Input: part model. Units: mm. Frame: model coordinates. Coordinates: 2 decimals unless noted, no trailing zeros. Loops run counter-clockwise (first coordinate to the right, second up) from the corner with the lowest first, then second, coordinate; pieces in that order, holes last.
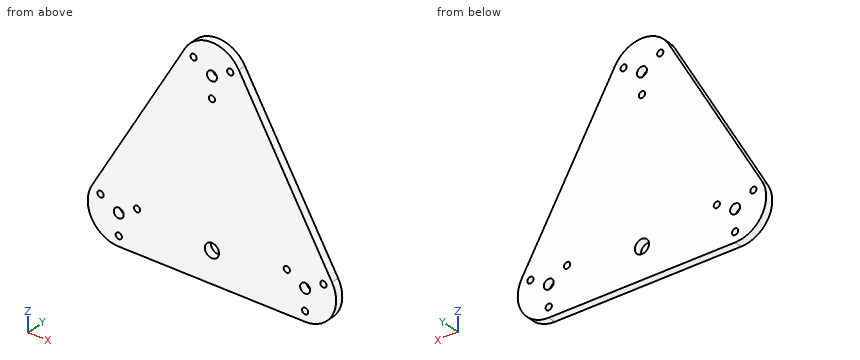
```python
from build123d import *

# Parameters (mm, degrees)
ESQUISSE1_R             = 5.7
ESQUISSE1_R_2           = 4
BOSS_EXTRU_1_DEPTH      = 6.35
ESQUISSE4_R             = 2.5
ENL_V_MAT_EXTRU_1_DEPTH = 6.35


with BuildPart() as part:
    # Esquisse1 → Boss.-Extru.1 (new body)
    with BuildSketch(Plane(origin=(0, 0, 0), x_dir=(1, 0, 0), z_dir=(0, 1, 0))):
        with BuildLine():
            Line((-96.654639651, 52.506938663), (-21.654639651, -77.493061337))
            ThreePointArc((-21.654639651, -77.493061337), (0, -90), (21.654639651, -77.493061337))
            Line((21.654639651, -77.493061337), (96.654639651, 52.506938663))
            ThreePointArc((96.654639651, 52.506938663), (96.648631983, 77.50346885), (75, 90))
            Line((75, 90), (-75, 90))
            ThreePointArc((-75, 90), (-96.648631983, 77.50346885), (-96.654639651, 52.506938663))
        make_face()
        with Locations(Location((0, 65, 0), (0, 0, 270))):
            Circle(ESQUISSE1_R, mode=Mode.SUBTRACT)
        with Locations(Location((-75, 65, 0), (0, 0, 270))):
            Circle(ESQUISSE1_R_2, mode=Mode.SUBTRACT)
        with Locations(Location((75, 65, 0), (0, 0, 270))):
            Circle(ESQUISSE1_R_2, mode=Mode.SUBTRACT)
        with Locations(Location((0, -65, 0), (0, 0, 270))):
            Circle(ESQUISSE1_R_2, mode=Mode.SUBTRACT)
    extrude(amount=BOSS_EXTRU_1_DEPTH)

    # Esquisse4 → Enlèv. mat.-Extru.1 (cut)
    with BuildSketch(Plane.XZ):
        with Locations(Location((-75, -82, 0), (0, 0, 90))):
            Circle(ESQUISSE4_R)
        with Locations(Location((-89.722431864, -56.5, 0), (0, 0, 90))):
            Circle(ESQUISSE4_R)
        with Locations(Location((-60.277568136, -56.5, 0), (0, 0, 90))):
            Circle(ESQUISSE4_R)
        with Locations(Location((60.277568136, -56.5, 0), (0, 0, 90))):
            Circle(ESQUISSE4_R)
        with Locations(Location((75, -82, 0), (0, 0, 90))):
            Circle(ESQUISSE4_R)
        with Locations(Location((89.722431864, -56.5, 0), (0, 0, 90))):
            Circle(ESQUISSE4_R)
        with Locations(Location((-14.722431864, 73.5, 0), (0, 0, 90))):
            Circle(ESQUISSE4_R)
        with Locations(Location((0, 48, 0), (0, 0, 90))):
            Circle(ESQUISSE4_R)
        with Locations(Location((14.722431864, 73.5, 0), (0, 0, 90))):
            Circle(ESQUISSE4_R)
    extrude(amount=-ENL_V_MAT_EXTRU_1_DEPTH, mode=Mode.SUBTRACT)


solid = part.part
```
Item 1: Section query A-A (z = -65). Output: boundary loops of the cut face in (x, y), then the cut area to 3 significant figures.
Result:
outline: (-100, 0) - (-79, 0) - (-79, 6.35) - (-100, 6.35) - close; (-71, 0) - (-5.7, 0) - (-5.7, 6.35) - (-71, 6.35) - close; (5.7, 0) - (71, 0) - (71, 6.35) - (5.7, 6.35) - close; (79, 0) - (100, 0) - (100, 6.35) - (79, 6.35) - close
area: 1,100 mm2
Item 2: Contact query for flat-ended pins moving along their axis: P1, Ø6, axis at x = 75, z = -82, coming from the +Y side; P2, Ø4.5, axis at x = 89.72, z = -56.5, coming from the -Y side; P3, Ø2, axis at y = 4.5, z = -50, coming from the +X side; P4, Ø3, axis at x = 13.5, y = 3, coming from the +Z side. Output: stop coordinate, or through.
Result:
P1: stops at y = 6.35
P2: passes through
P3: stops at x = 95.79
P4: stops at z = 86.93
Item 3: Section query B-B (z = 65). Output: boundary loops of the cut face in (x, y).
Result:
outline: (-28.86, 0) - (-4, 0) - (-4, 6.35) - (-28.86, 6.35) - close; (4, 0) - (28.86, 0) - (28.86, 6.35) - (4, 6.35) - close
Item 4: Line query: L1, parallel to X at y = 5, z = -65; L2, parallel to X at y = 1.75, z = -66; L3, parallel to X at y = 3.75, z = -56.5. Output: solid intervals per line, ascending.
Result:
L1: x = -100 to -79, -71 to -5.7, 5.7 to 71, 79 to 100
L2: x = -99.98 to -78.87, -71.13 to -5.61, 5.61 to 71.13, 78.87 to 99.98
L3: x = -98.51 to -92.22, -87.22 to -62.78, -57.78 to 57.78, 62.78 to 87.22, 92.22 to 98.51
Item 5: Section query C-C (y = 1). Count the separate pieces of the cut face and the enclosed holes in it, then the cut area to 3 significant figures.
Result:
separate pieces: 1
enclosed holes: 13
area: 22,500 mm2
Item 6: Section query D-D (x = -52.5). Output: boundary loops of the cut face in (y, z), then the cut area to 3 significant figures.
Result:
outline: (0, -90) - (6.35, -90) - (6.35, 24.03) - (0, 24.03) - close
area: 724 mm2
